```python
from build123d import *

# Parameters (mm, degrees)
F0_R     = 38.1
F1_DEPTH = 25.4
F2_R     = 5.08
F3_W     = 19.05
F3_H     = 19.05
F4_DEPTH = 25.401
F5_R     = 5.08


with BuildPart() as f1:
    # F0 (on Front) → F1 (new body)
    with BuildSketch(Plane.XZ):
        Circle(F0_R)
    extrude(amount=F1_DEPTH)

    # F2
    f2_edges = [f1.edges().sort_by_distance(p)[0] for p in [
        (-38.1, -25.4, 0),
    ]]
    fillet(f2_edges, radius=F2_R)

    # F3 (on face) → F4 (cut, through all)
    with BuildSketch(Plane(origin=(0, 0, 0), x_dir=(-1, 0, 0), z_dir=(0, 1, 0))):
        Rectangle(F3_W, F3_H)
    extrude(amount=-F4_DEPTH, mode=Mode.SUBTRACT)

    # F5
    f5_edges = [f1.edges().sort_by_distance(p)[0] for p in [
        (0, -25.4, 9.525),
        (-9.525, -25.4, 0),
        (0, -25.4, -9.525),
        (9.525, -25.4, 0),
    ]]
    fillet(f5_edges, radius=F5_R)


solid = f1.part
```
For this review, take the finished solid that the model builds, in its own axes (mm). A direction names the side the tool comes from. Coordinates: 2 decimals unless noted, no trailing zeros. Order: outer loops, then holes, each group sorted by start corner. A loop starts at its lowest first (then second) coordinate and runs counter-clockwise, first axis right, second up. Notation, with made-up numbers: (45, -19) -> (53, -19) arc R31 cw to (53, 10) -> close; hole circle Ø10 at (22, -18). An arc over 180 degrees is marked (long way). Use CSV: the item, a comma, the result in double quotes. Start each with the question number.
Item 1: We need section D-D, the plane y = -23. Give the boundary of the cut face in (x, z).
Item 2: We need section A-A, the plane z = 0. Give the boundary of the cut face in (x, y) (3 decimals), then the cut area to 3 significant figures.
Item 3: For faces 5 (the face through (9.525, -10, 0)), 6 (the face through (-15, -25.4, 0)), 7 (the face through (0.2, -23.95, -11.05)), list the 3-axis set-ups (+Z, -Z, +X, -X, +Y, -Y) from which the entire face can be reached by the end or side of a thin tool; tool diameter is ignored.
Item 4: We need section B-B, the plane x = 0. Give the boundary of the cut face in (y, z) (3 decimals), then the cut area to 3 significant figures.
Item 5: Draft analysis for pull direction Z (two halves, no side actions). For faces 1 (the face through (-11.05, -23.95, -0.2)), 2 (the face through (-30.235, -10.018, -23.183)), 3 (the face through (16, 0, 1)), 4 (the face through (0.2, -23.95, 11.05)), state which applies: pulls with the +Z half, pulls with the -Z half, needs draft (parallel to the pull), parting line crosses it, or undercut.
Item 6: Wall thickness on probe 1 along Z at (x, y) = (-1, -4) (3 decimals); probe 2 along X at (y, z) = (-2.75, -9) (3 decimals); probe 3 along X at (y, z) = (-5, 5.5) (3 decimals): over which ranges is each line inside the solid? List them lowest first.
Item 7: Insertion check: pin 1 (10 mm diameter, centred on y = -14, z = 17, fed in from -X); pin 2 (12 mm diameter, centred on x = 12.5, y = -2.5, fed in from +Z); pin 3 (6 mm diameter, centred on y = -14, z = -4.5, fed in from +X). Each pin has a flat end and moves straight along its axis. Give the tip position at first contact, or say it passes through.
Item 8: We need section C-C, the plane y = -9.5. Give the boundary of the cut face in (x, z) (3 decimals).
Derived:
1,outline,"circle Ø74.67 at (0, 0); hole (-10.29, -10.29) -> (10.29, -10.29) -> (10.29, 10.29) -> (-10.29, 10.29) -> close"
2,outline,"(-38.1, -20.32) arc R5.08 ccw to (-33.02, -25.4) -> (-14.605, -25.4) arc R5.08 ccw to (-9.525, -20.32) -> (-9.525, 0) -> (-38.1, 0) -> close; (9.525, -20.32) arc R5.08 ccw to (14.605, -25.4) -> (33.02, -25.4) arc R5.08 ccw to (38.1, -20.32) -> (38.1, 0) -> (9.525, 0) -> close"
2,area,"1,430 mm^2"
3,face 5,"+Y, -Y"
3,face 6,"+Z, -Z, +X, -X, -Y"
3,face 7,"-Y"
4,outline,"(-25.4, -33.02) arc R5.08 ccw to (-20.32, -38.1) -> (0, -38.1) -> (0, -9.525) -> (-20.32, -9.525) arc R5.08 ccw to (-25.4, -14.605) -> close; (-25.4, 14.605) arc R5.08 ccw to (-20.32, 9.525) -> (0, 9.525) -> (0, 38.1) -> (-20.32, 38.1) arc R5.08 ccw to (-25.4, 33.02) -> close"
4,area,"1,430 mm^2"
5,face 1,"undercut"
5,face 2,"parting line crosses it"
5,face 3,"needs draft"
5,face 4,"undercut"
6,probe 1,"z = -38.087 to -9.525, 9.525 to 38.087"
6,probe 2,"x = -37.022 to -9.525, 9.525 to 37.022"
6,probe 3,"x = -37.701 to -9.525, 9.525 to 37.701"
7,pin 1,"stops at x = -36.16"
7,pin 2,"stops at z = 37.54"
7,pin 3,"stops at x = 38.07"
8,outline,"circle Ø76.2 at (0, 0); hole (-9.525, -9.525) -> (9.525, -9.525) -> (9.525, 9.525) -> (-9.525, 9.525) -> close"
